Autodesk Inventor part; units mm, degrees
ref_plane "Work Plane1" through (0, 0, 67.5) normal (0, 0, 1) x (1, 0, 0)
ref_plane "Work Plane3" through (-30, 0, 94) normal (0, -0.4226, 0.9063) x (1, 0, 0)
ref_plane "YZ Plane" through (0, 0, 0) normal (1, 0, 0) x (0, 1, 0)
sketch "Sketch1" plane through (0, 0, 0) normal (0, 0, 1) x (1, 0, 0)
  circle A0 centre (0, 0) radius 40
  circle A1 centre (0, 0) radius 30
  dimension "d0" = 80
  dimension "d1" = 60
extrude "Extrusion1" add sketch "Sketch1" along normal blind 135
sketch "Sketch2" plane through (0, 0, 135) normal (0, 0, 1) x (1, 0, 0)
  circle A0 centre (0, 0) radius 65
  circle A1 centre (0, 0) radius 30
  dimension "d4" = 130
extrude "Extrusion2" add sketch "Sketch2" along normal blind 14
sketch "Sketch3" plane through (0, 0, 0) normal (0, 0, -1) x (-1, 0, 0)
  point P0 (0, 0)
sketch "Sketch4" plane through (0, 0, 149) normal (0, 0, 1) x (1, 0, 0)
  circle A0 centre (0, 0) radius 50
  circle A1 centre (-50, 0) radius 5
  circle A2 centre (0, -50) radius 5
  circle A3 centre (50, 0) radius 5
  circle A4 centre (0, 50) radius 5
  dimension "d7" = 100
  dimension "d8" = 10
  dimension "d11" = 360
extrude "Extrusion3" cut sketch "Sketch4" against normal blind 14 contours A0 A3 | A0 A3 | A4 A0 | A0 A4 | A2 A0 | A0 A2 | A1 A0 | A0 A1
ref_plane "Work Plane1" through (0, 0, 67.5) normal (0, 0, 1) x (1, 0, 0)
mirror "Mirror1" about plane through (0, 0, 67.5) normal (0, 0, 1) of "Extrusion2", "Extrusion3"
ref_plane "Work Plane2" through (0, 0, 94) normal (0, 0, 1) x (1, 0, 0)
sketch "Sketch5" plane through (0, 0, 94) normal (0, 0, 1) x (1, 0, 0)
  circle A0 centre (0, 0) radius 30
  line L0 (-30, 0) -> (30, 0)
ref_plane "Work Plane3" through (-30, 0, 94) normal (0, -0.4226, 0.9063) x (1, 0, 0)
sketch "Sketch6" plane through (0, 0, 0) normal (1, 0, 0) x (0, 1, 0)
  point P0 (0, 0)
sketch "Sketch7" plane through (-30, 0, 94) normal (0, -0.4226, 0.9063) x (1, 0, 0)
  point P0 (30, -39.7261)
sketch "Sketch8" plane through (-30, 0, 94) normal (0, -0.4226, 0.9063) x (1, 0, 0)
  point P0 (30, -39.7261)
sketch "Sketch9" plane through (0, 0, 94) normal (0, 0, 1) x (1, 0, 0)
  point P0 (0, 0)
sketch "Sketch10" plane through (-30, 0, 94) normal (0, -0.4226, 0.9063) x (1, 0, 0)
  point P0 (30, -39.7261)
sketch "Sketch11" plane through (0, 0, 0) normal (1, 0, 0) x (0, 1, 0)
  line L0 (5, -14) -> (-5, -14) construction
  line L1 (0, -14) -> (0, 41) construction
  line L2 (0, 41) -> (115.1011, 94.6725) construction
  point P0 (0, 0)
  dimension "d18" = 127
  dimension "d19" = 115
  dimension "d20" = 55
ref_plane "Work Plane4" through (0, 115.1011, 94.6725) normal (0, 0.9063, 0.4226) x (-1, 0, 0)
sketch "Sketch12" plane through (0, 115.1011, 94.6725) normal (0, 0.9063, 0.4226) x (-1, 0, 0)
  circle A0 centre (0, 0) radius 30
  circle A1 centre (0, 0) radius 25
  point P0 (0, -37.1586)
  dimension "d21" = 60
  dimension "d22" = 50
extrude "Extrusion4" add sketch "Sketch12" against normal up to next
sketch "Sketch13" plane through (0, 115.1011, 94.6725) normal (0, 0.9063, 0.4226) x (1, 0, 0)
  line L0 (54.3855, -57.451) -> (-55.6145, -57.451)
  line L1 (-64.2747, -42.451) -> (-9.2747, 52.8118)
  line L2 (8.0458, 52.8118) -> (63.0458, -42.451)
  arc A0 (54.3855, -57.451) -> (63.0458, -42.451) centre (54.3855, -47.451) ccw
  arc A1 (-64.2747, -42.451) -> (-55.6145, -57.451) centre (-55.6145, -47.451) ccw
  arc A2 (8.0458, 52.8118) -> (-9.2747, 52.8118) centre (-0.6145, 47.8118) ccw
  line L3 (54.3855, -47.451) -> (-55.6145, -47.451) construction
  circle A3 centre (54.3855, -47.451) radius 5
  circle A4 centre (-55.6145, -47.451) radius 5
  circle A5 centre (-0.6145, 47.8118) radius 5
  line L4 (-0.6145, -57.451) -> (-0.6145, -2.451) construction
  point P0 (0, 37.1586)
  dimension "d25" = 10
  dimension "d26" = 110
  dimension "d28" = 10
  dimension "d29" = 10
  dimension "d30" = 10
  dimension "d31" = 55
extrude "Extrusion5" add sketch "Sketch13" along normal blind 10 and the other way blind 5
sketch "Sketch14" plane through (0, 124.1642, 98.8987) normal (0, 0.9063, 0.4226) x (1, 0, 0)
  circle A0 centre (0, 0) radius 25
  circle A1 centre (0, 0) radius 30
  point P0 (0, 37.1586)
extrude "Extrusion6" cut sketch "Sketch14" against normal blind 10 contours A0 | A1
sketch "Sketch15" plane through (0, 115.1011, 94.6725) normal (0, 0.9063, 0.4226) x (1, 0, 0)
  circle A0 centre (0, 0) radius 30
  circle A1 centre (0, 0) radius 25
  point P0 (0, 37.1586)
  dimension "d38" = 50
extrude "Extrusion7" cut sketch "Sketch15" against normal blind 120 contours A1
properties part number "cad@63"
Part model, mm, in its own coordinate system. A direction names the side the tool comes from. Round coordinates to 2 decimals unless told otherwise and drop trailing zeros. Answer as a JSON object with one key per item and string values.
Item 1: Pull direction Z, two halves, no side cores. Call faces 1 (the face through (-1.52, 108.34, 132.83)), 2 (the face through (59.155, 96.583, 140.051)), 3 (the face through (45, 0, -7)): pulls with the +Z half, pulls with the -Z half, needs draft (parallel to the pull), parting line crosses it, or undercut.
Output:
{"face 1": "pulls with the +Z half", "face 2": "undercut", "face 3": "needs draft"}
Item 2: Pin check, flat tips, straight feed: pin 1 (10 mm diameter, centred on y = 35, z = 118.5, fed in from -X); pin 2 (8 mm diameter, centred on x = 50, y = 0, fed in from -Z); pin 3 (13 mm diameter, centred on x = 0, y = 50, fed in from -Z); pin 4 (10 mm diameter, centred on y = -21, z = 27, fed in from +X). Stop position of each tip, or through.
Output:
{"pin 1": "x = -26.46", "pin 2": "through", "pin 3": "z = -14", "pin 4": "x = 36.66"}
Item 3: Tool access for faces 4 (the face through (-0.651, -54.957, -7.098)), 5 (the face through (-0.651, 54.957, 142.098)), 6 (the face through (-28, 30, 0)): list every direction of +Z, -Z, +X, -X, +Y, -Y with a clear straight run to the whole face (end or side of a thin tool).
Output:
{"face 4": "+Z, -Z", "face 5": "+Z", "face 6": "none"}
Item 4: Band-saw the part on A-A on y = 0. State how many separate pieces and enclosed holes the cut face has, plus the area to 3 significant figures.
Output:
{"separate pieces": "6", "enclosed holes": "0", "area": "4,100 mm2"}
Item 5: Wall check: L1, parallel to Y at x = 0, z = -7; L2, parallel to Z at x = -40.5, y = -9; L3, parallel to Z at x = -14, y = 98. Give the ranges that are in metal, low to high.
Output:
{"L1": "-65 to -55, -45 to -30, 30 to 45, 55 to 65", "L2": "-14 to 0, 135 to 149", "L3": "57.42 to 63.84, 109.55 to 115.97, 119.51 to 150.09"}
